```python
from build123d import *

# Parameters (mm, degrees)
BOSS_EXTRUDE2_DEPTH = 35
SKETCH6_R           = 1.27
CUT_EXTRUDE2_DEPTH  = 21
CUT_EXTRUDE3_DEPTH  = 14


with BuildPart() as part:
    # Sketch1 → Boss-Extrude2 (new body)
    with BuildSketch(Plane(origin=(0, 0, 0), x_dir=(1, 0, 0), z_dir=(0, 1, 0))):
        Polygon((3.521836642, 6.1), (-3.521836642, 6.1), (-7.043673284, 0), (-3.521836642, -6.1), (3.521836642, -6.1), (7.043673284, 0), align=None)
    extrude(amount=BOSS_EXTRUDE2_DEPTH)

    # Sketch6 → Cut-Extrude2 (cut)
    with BuildSketch(Plane.XZ):
        Circle(SKETCH6_R)
    extrude(amount=-CUT_EXTRUDE2_DEPTH, mode=Mode.SUBTRACT)

    # Sketch7 → Cut-Extrude3 (cut)
    with BuildSketch(Plane(origin=(0, 35, 0), x_dir=(1, 0, 0), z_dir=(0, 1, 0))):
        with BuildLine():
            Line((-1.322875656, 1.5), (1.322875656, 1.5))
            ThreePointArc((1.322875656, 1.5), (0, -2), (-1.322875656, 1.5))
        make_face()
    extrude(amount=-CUT_EXTRUDE3_DEPTH, mode=Mode.SUBTRACT)


solid = part.part
```
Check sheet for the modelled part. Datum: model origin and axes. Units: mm. A direction names the side the tool comes from. Coordinates: 2 decimals unless noted, no trailing zeros. Write each loop counter-clockwise with the first axis right and the second up, starting at its lowest first coordinate (ties: lowest second). Pieces come first, ordered by that corner, then holes. Notation, with made-up numbers: M 70,76.25 L 110,76.25 A22 ccw 110,87.25 Z; hole C -38.75,71.25 d4. An arc over 180 degrees is marked long. Use one line per item in the form item = value.
Item 1: Sectioned sample at C-C, the plane z = -0.75. Record the cut outline in (x, y).
Answer below:
outline = M -6.61,0 L -1.02,0 L -1.02,21 L -1.85,21 L -1.85,35 L -6.61,35 Z; M 1.02,0 L 6.61,0 L 6.61,35 L 1.85,35 L 1.85,21 L 1.02,21 Z
Item 2: Material ranges on L1, parallel to Z at x = 0, y = 12; L2, parallel to Z at x = -0.5, y = 10; L3, parallel to X at y = 23.5, z = 5.25, recorded low to high. Write a range as from..to.
Answer below:
L1 = -6.1..-1.27, 1.27..6.1
L2 = -6.1..-1.17, 1.17..6.1
L3 = -4.01..4.01
Item 3: Release check for a two-part mould opening along X. For faces 3 (the face through (0, 28, 2)), 4 (the face through (1.5, 0, -0.1)), 5 (the face through (-5.26, 17.26, -3.09)) record: pulls with the +X half, pulls with the -X half, needs draft (parallel to the pull), parting line crosses it, or undercut.
Answer below:
face_3 = undercut
face_4 = needs draft
face_5 = pulls with the -X half
Item 4: Gauge pin test, flat ends, axial feed: pin 1 Ø1.8 at (x, z) = (-0.5, 0) entering from +Y; pin 2 Ø6 at (y, z) = (6, 4.5) entering from -X; pin 3 Ø4 at (y, z) = (12.5, 0.5) entering from +X. Record the tip position at first contact, or that the pin passes through.
Answer below:
pin_1 = 21
pin_2 = -6.18
pin_3 = 7.04
Item 5: Sectioned sample at A-A, the plane x = 0. Record the cut outline in (y, z), and give its area (3 significant figures).
Answer below:
outline = M 0,-6.1 L 35,-6.1 L 35,-1.5 L 21,-1.5 L 21,-1.27 L 0,-1.27 Z; M 0,1.27 L 21,1.27 L 21,2 L 35,2 L 35,6.1 L 0,6.1 Z
area = 325 mm^2
Item 6: Sectioned sample at D-D, the plane y = 15. Record the cut outline in (x, z), and give its area (3 significant figures).
Answer below:
outline = M -7.04,0 L -3.52,-6.1 L 3.52,-6.1 L 7.04,0 L 3.52,6.1 L -3.52,6.1 Z; hole C 0,0 d2.54
area = 124 mm^2
Item 7: Set-up check for faces 1 (the face through (0, 28, -1.5)), 2 (the face through (5.307, 17.255, -3.007)): record each of +Z, -Z, +X, -X, +Y, -Y from which the full face is reachable in a straight line by a thin tool's end or side.
Answer below:
face_1 = +Y
face_2 = -Z, +X, +Y, -Y
Item 8: Sectioned sample at B-B, the plane y = 23.5. Record the cut outline in (x, z).
Answer below:
outline = M -7.04,0 L -3.52,-6.1 L 3.52,-6.1 L 7.04,0 L 3.52,6.1 L -3.52,6.1 Z; hole M -1.32,-1.5 L 1.32,-1.5 A2 ccw long Z
